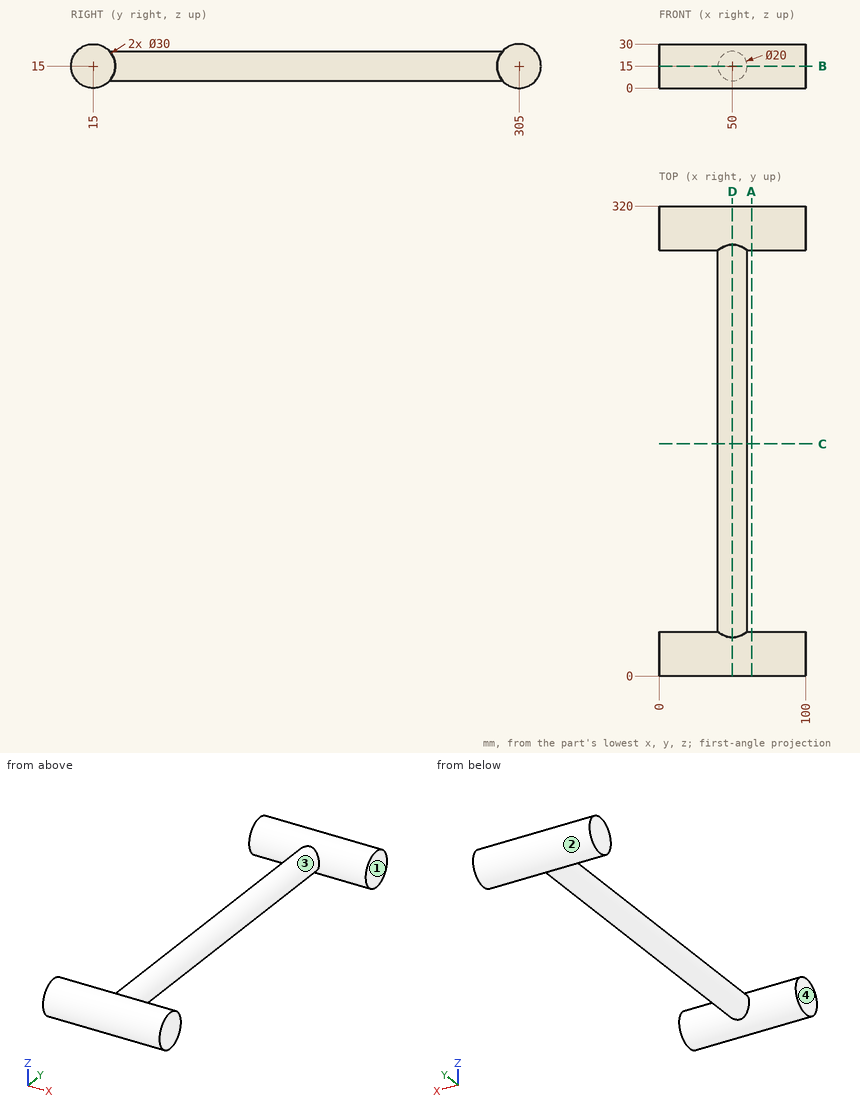
Job drawing, mm, ordinate dimensions from the low corner. One solid piece. A direction names the side the tool comes from. Give positions to 0.01 mm unless a question says otherwise; leave off trailing zeros. Order: outer loops, then holes, each group sorted by start corner. A loop starts at its lowest first (then second) coordinate and runs counter-clockwise, first axis right, second up. Notation, with made-up numbers: (71.5, 57) - (119.5, 57) arc R22 cw to (119.5, 95) - close; hole circle Ø5 at (62.5, -20.75). An arc over 180 degrees is marked (long way). Return JSON: item names as keys, results as strings.
1) Cut at A-A, the plane x = 63. Give the cut face in (y, z).
Geometry says:
{"outline": "circle Ø30 at (15, 15); circle Ø30 at (305, 15)"}
2) Cut at D-D, the plane x = 50. Give the cut face in (y, z).
Geometry says:
{"outline": "(26.18, 5) - (293.82, 5) arc R15 ccw (long way) to (293.82, 25) - (26.18, 25) arc R15 ccw (long way) to start"}
3) Flat gauge pins, fed straight in: P1, Ø2, axis at x = 58, y = 226, coming from the +Z side; P2, Ø1, axis at y = 183.5, z = 20.5, coming from the -X side; P3, Ø3, axis at y = 273.5, z = 3, coming from the -X side; P4, Ø8, axis at x = 55.5, y = 238, coming from the -Z side. Where does each tip first touch, or does it go through?
Geometry says:
{"P1": "z = 22.14", "P2": "x = 41.34", "P3": "through", "P4": "z = 5.11"}
4) Pull direction Y, two halves, no side cores. Call the marked faces 1 and 2: pulls with the +Y half, pulls with the -Y half, needs draft (parallel to the pull), parting line crosses it, or undercut.
Geometry says:
{"face 1": "needs draft", "face 2": "undercut"}
5) 3-axis set-ups, long thin cutter, end or side, ignore diameter. For the marked faces 3 and 4: which of +Z, -Z, +X, -X, +Y, -Y reach the whole face in a straight line?
Geometry says:
{"face 3": "none", "face 4": "+Z, -Z, -X, +Y, -Y"}
6) Cut at B-B, the plane z = 15. Give the cut face in (x, y).
Geometry says:
{"outline": "(0, 0) - (100, 0) - (100, 30) - (60, 30) - (60, 290) - (100, 290) - (100, 320) - (0, 320) - (0, 290) - (40, 290) - (40, 30) - (0, 30) - close"}
7) Probe line 1 (Y direction, x = 12, z = 15); line 2 (Y direction, x = 36, z = 12); line 3 (Y direction, x = 50, z = 15). List the from-to ranges inside material, lowest first. Write a range as from..to.
Geometry says:
{"line 1": "0..30, 290..320", "line 2": "0.3..29.7, 290.3..319.7", "line 3": "0..320"}
8) Cut at C-C, the plane y = 158. Give the cut face in (x, z), plus the area to 3 significant figures.
Geometry says:
{"outline": "circle Ø20 at (50, 15)", "area": "314 mm²"}
